Source: CAD feature listing. Evaluate the final solid. Frame: model axes, mm. Face numbers are marked on the shaded views. A direction names the side the tool comes from. Round coordinates to 2 decimals unless told otherwise and drop trailing zeros. Write each loop counter-clockwise with the first axis right and the second up, starting at its lowest first coordinate (ties: lowest second). Pieces come first, ordered by that corner, then holes. Notation, with made-up numbers: M 11,-2.75 L 33,-2.75 A26 ccw 33,21.25 Z; hole C 45,34.25 d8. An arc over 180 degrees is marked long. Answer in a Markdown table with one row per item. Add a question column.
Item 1: Cut plane D-D on x = -1. Return loops of the section in (y, z).
Item 2: Cut plane B-B on z = 8. Give the number of separate pieces and of enclosed holes in the cut face, and give its area (3 significant figures).
Item 3: Contact query for flat-ended pins moving along their axis: pin 1 (4 mm diameter, centred on x = -1, y = 15.05, fed in from +Z); pin 2 (2 mm diameter, centred on x = -1, y = 15.5, fed in from -Z). Output: stop coordinate, or through.
Item 4: Mould query, pull axis X, two halves, no side actions, for the marked faces 5, 6, 7 and 8. Classes: released by +X, released by -X, zero draft, split by the parting line, or undercut.
Item 5: Material intervals for probe 1 along Y at (x, z) = (-10, 3.75); probe 2 along X at (y, z) = (13.5, 8); probe 3 along X at (y, z) = (16.25, 15.5), sorted ascending.
Item 6: Set-up query: the marked faces 1, 2, 3 and 4. Return all of +Z, -Z, +X, -X, +Y, -Y with unobstructed straight access to the full face (end or side cutting, diameter ignored); none if empty.
Item 7: Cut plane A-A on x = -5.5. Return loops of the section in (y, z).
Autodesk Inventor part; units mm, degrees
ref_plane "РабПлоскость1" through (0, 0, 10) normal (0, 0, -1) x (-1, 0, 0)
ref_plane "YZ Plane" through (0, 0, 0) normal (1, 0, 0) x (0, 1, 0)
ref_plane "XZ Plane" through (0, 0, 0) normal (0, 1, 0) x (-1, 0, 0)
sketch "Эскиз1" plane through (0, 0, 0) normal (0, 0, 1) x (1, 0, 0)
  line L0 (13.5, 19.05) -> (-13.5, 19.05) construction
  circle A0 centre (-7.5, -8) radius 1.6 construction
  circle A1 centre (7.5, -8) radius 1.6 construction
  line L1 (-13.5, 19.05) -> (2.5, 19.05)
  line L2 (-13.5, 19.05) -> (-13.5, 9.05)
  line L3 (-13.5, 11.05) -> (2.5, 11.05)
  line L4 (-13.5, 11.05) -> (-13.5, 9.05)
  line L5 (2.5, 11.05) -> (2.5, 19.05)
  point P0 (2.5, 15.05)
  dimension "d3" = 0
  dimension "d15" = 16
extrude "Выдавливание1" add sketch "Эскиз1" along normal blind 20
ref_plane "РабПлоскость1" through (0, 0, 10) normal (0, 0, -1) x (-1, 0, 0)
sketch "Эскиз4" plane through (0, 0, 20) normal (0, 0, 1) x (1, 0, 0)
  line L0 (2.5, 11.05) -> (2.5, 19.05) construction
  line L1 (2.5, 15.05) -> (-13.5, 15.05) construction
  line L2 (-13.5, 19.05) -> (-13.5, 11.05) construction
  circle A0 centre (-10, 15.05) radius 2.1
  circle A1 centre (-1, 15.05) radius 2.1
  point P0 (0, 0)
  point P1 (-13.5, 9.05)
  dimension "d16" = 4.2
  dimension "d17" = 4.2
  dimension "d18" = 3.5
  dimension "d19" = 3.5
extrude "Выдавливание4" cut sketch "Эскиз4" against normal blind 5
mirror "Зеркальное отражение2" about plane through (0, 0, 10) normal (0, 0, -1) of "Выдавливание4"
sketch "Эскиз5" plane through (-13.5, 19.05, 0) normal (0, 1, 0) x (1, 0, 0)
  line L0 (16, 0) -> (0, 0) construction
  line L1 (0, 0) -> (0, -20) construction
  line L2 (16, -20) -> (0, -20) construction
  line L3 (16, 0) -> (16, -20) construction
  line L4 (8, -7.407) -> (8, -12.593) construction
  line L5 (6.5, -7.407) -> (6.5, -12.593)
  line L6 (9.5, -12.593) -> (9.5, -7.407)
  arc A0 (9.5, -7.407) -> (6.5, -7.407) centre (8, -7.407) ccw
  arc A1 (6.5, -12.593) -> (9.5, -12.593) centre (8, -12.593) ccw
  point P0 (13.5, 0)
  point P1 (8, -10)
  dimension "d22" = 3
extrude "Выдавливание5" cut sketch "Эскиз5" against normal blind 20
ref_plane "РабПлоскость2" through (0, 0, 10) normal (0, 0, 1) x (1, 0, 0)
sketch "Эскиз7" plane through (0, 0, 10) normal (0, 0, 1) x (1, 0, 0)
  line L0 (-7, 19.05) -> (-7, 11.05) construction
  arc A0 (-13.5, 11.05) -> (-12.8908, 11.202) centre (-15.1731, 19.05) ccw
  arc A1 (-7, 19.55) -> (-7.0153, 18.5502) centre (-7, 19.05) ccw construction
  line L1 (-7, 19.05) -> (-7, 19.55) construction
  arc A2 (-7, 16.629) -> (-7.1382, 17.5535) centre (-7.2447, 17.065) ccw
  arc A3 (-7.7422, 15.6469) -> (-8.2131, 14.7653) centre (-7.9642, 15.1989) ccw construction
  arc A4 (-8.7912, 13.9441) -> (-9.4621, 13.2033) centre (-9.1153, 13.5634) ccw construction
  arc A5 (-10.2223, 12.547) -> (-11.0531, 11.9913) centre (-10.6292, 12.2564) ccw construction
  arc A6 (-11.9499, 11.5393) -> (-12.8908, 11.202) centre (-12.4152, 11.3563) ccw construction
  arc A7 (-7, 18.55) -> (-6.5, 19.05) centre (-7, 19.05) ccw
  arc A8 (-7.3809, 16.5839) -> (-7, 16.629) centre (-7.2447, 17.065) ccw
  arc A9 (-7.1382, 17.5535) -> (-7.3809, 16.5839) centre (-7.2447, 17.065) ccw construction
  arc A10 (-8.2131, 14.7653) -> (-7.7422, 15.6469) centre (-7.9642, 15.1989) ccw
  arc A11 (-9.4621, 13.2033) -> (-8.7912, 13.9441) centre (-9.1153, 13.5634) ccw
  arc A12 (-11.0531, 11.9913) -> (-10.2223, 12.547) centre (-10.6292, 12.2564) ccw
  arc A13 (-12.8908, 11.202) -> (-11.9499, 11.5393) centre (-12.4152, 11.3563) ccw
  line L2 (-4, 11.05) -> (-7, 11.05)
  arc A14 (-7.0153, 18.5502) -> (-7, 19.05) centre (-15.1731, 19.05) ccw construction
  arc A15 (-7.1382, 17.5535) -> (-7.0153, 18.5502) centre (-15.1731, 19.05) ccw
  arc A16 (-7.7422, 15.6469) -> (-7.3809, 16.5839) centre (-15.1731, 19.05) ccw
  arc A17 (-7.3809, 16.5839) -> (-7.1382, 17.5535) centre (-15.1731, 19.05) ccw construction
  arc A18 (-8.2131, 14.7653) -> (-7.7422, 15.6469) centre (-15.1731, 19.05) ccw construction
  arc A19 (-8.7912, 13.9441) -> (-8.2131, 14.7653) centre (-15.1731, 19.05) ccw
  arc A20 (-9.4621, 13.2033) -> (-8.7912, 13.9441) centre (-15.1731, 19.05) ccw construction
  arc A21 (-11.0531, 11.9913) -> (-10.2223, 12.547) centre (-15.1731, 19.05) ccw construction
  arc A22 (-11.9499, 11.5393) -> (-11.0531, 11.9913) centre (-15.1731, 19.05) ccw
  arc A23 (-12.8908, 11.202) -> (-11.9499, 11.5393) centre (-15.1731, 19.05) ccw construction
  arc A24 (-10.2223, 12.547) -> (-9.4621, 13.2033) centre (-15.1731, 19.05) ccw
  arc A25 (-13.5, 12.2806) -> (-8.2, 19.05) centre (-15.1731, 19.05) ccw
  line L3 (-8.2, 19.05) -> (-6.5, 19.05)
  line L4 (2.5, 19.05) -> (-13.5, 19.05)
  line L5 (-13.5, 19.05) -> (-13.5, 11.05)
  line L6 (-13.5, 11.05) -> (-13.5, 12.2806)
  arc A26 (-7.0153, 18.5502) -> (-7, 18.55) centre (-7, 19.05) ccw
  line L7 (-13.5, 11.05) -> (-12.4152, 10.8563)
  point P0 (0, 0)
  point P1 (-7, 19.05)
  point P2 (-7.0153, 18.5502)
  dimension "d25" = 1
  dimension "d34" = 1
  dimension "d36" = 1
  dimension "d39" = 1
  dimension "d40" = 1
  dimension "d41" = 1
  dimension "d42" = 1
  dimension "d43" = 1
  dimension "d44" = 1
  dimension "d45" = 1
  dimension "d46" = 1
  dimension "d48" = 1.2
extrude "Выдавливание6" cut sketch "Эскиз7" along normal blind 12 and the other way blind 3 contours L5 A25 L3 A7 A26 A15 A2 A8 A16 A10 A19 A11 A24 A12 A22 A13 L7 A0 | A0 A13 L7
properties part number "стена_каретки" material "Полипропилен"
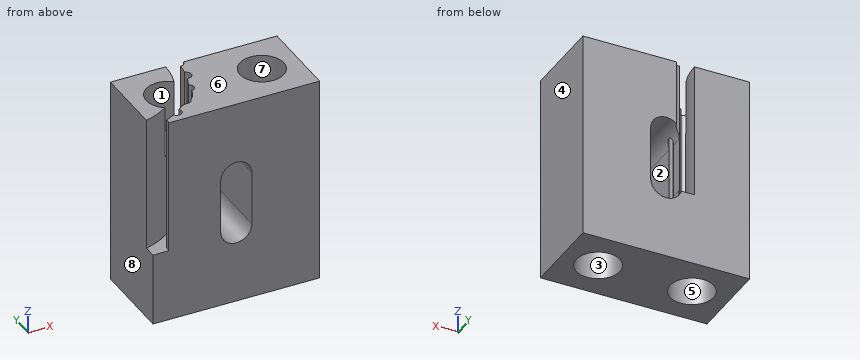
Results below:
| question | item | result |
|---|---|---|
| 1 | outline | M 11.05,0 L 12.95,0 L 12.95,5 L 17.15,5 L 17.15,0 L 19.05,0 L 19.05,20 L 17.15,20 L 17.15,15 L 12.95,15 L 12.95,20 L 11.05,20 Z |
| 2 | separate pieces | 4 |
| 2 | enclosed holes | 0 |
| 2 | area | 90.0 mm2 |
| 3 | pin 1 | z = 15 |
| 3 | pin 2 | z = 5 |
| 4 | face 5 | undercut |
| 4 | face 6 | zero draft |
| 4 | face 7 | undercut |
| 4 | face 8 | released by -X |
| 5 | probe 1 | 11.05 to 12.95, 17.15 to 19.05 |
| 5 | probe 2 | -13.5 to -10.95, -8.62 to -7, -4 to 2.5 |
| 5 | probe 3 | -13.5 to -11.72, -7.49 to -2.72, 0.72 to 2.5 |
| 6 | face 1 | +Z |
| 6 | face 2 | +Y, -Y |
| 6 | face 3 | -Z |
| 6 | face 4 | +Z, -Z, +X, +Y, -Y |
| 7 | outline | M 11.05,0 L 19.05,0 L 19.05,5.91 L 11.05,5.91 Z; M 11.05,14.09 L 19.05,14.09 L 19.05,20 L 11.05,20 Z |
